CAD build for the part. Positions are in the model's coordinates, mm. A direction names the side the tool comes from. Round coordinates to 2 decimals unless told otherwise and drop trailing zeros. Write each loop counter-clockwise with the first axis right and the second up, starting at its lowest first coordinate (ties: lowest second). Pieces come first, ordered by that corner, then holes. Notation, with made-up numbers: (89, 71.25) - (126, 71.25) arc R16 ccw to (126, 77.25) - close; hole circle Ø8 at (-34, 81). An arc over 180 degrees is marked (long way). Put each result on its own line as item: value. Start each with the question number.
Item 1: Cut at C-C (z = 12.75). Give the cut face in (x, y).
Item 2: Cut at A-A (x = 40). Give the cut face in (y, z), and give its area (3 significant figures).
Item 3: 3-axis set-ups, long thin cutter, end or side, ignore diameter. For faces 1 (the cylindrical face through (9.1, 19.5, 8.8)), 2 (the flat face through (49, 10, 1)): which of +Z, -Z, +X, -X, +Y, -Y reach the whole face in a straight line?
Item 4: Pin check, flat tip, straight feed: pin 1 Ø5 at (x, z) = (30, 10) entering from +Y. Stop position of the tip, or through.
Item 5: Mould opens along Z. For faces 3 (the cylindrical face through (86.15, 15.07, 0.51)), 4 (the cylindrical face through (61.487, 19.507, 9.805)) say: released by +Z, released by -Z, zero draft, split by the parting line, or undercut.
Item 6: Cut at B-B (y = 5). Give the cut face in (x, z), and give its area (3 significant figures).
Item 7: Drill centre lines: line 1 (Y direction, x = 87.65, z = 19.45); line 2 (Y direction, x = 25.5, z = 7.5). Where is each one in solid material? Low to high. Write a range as from..to.
```python
from build123d import *

# Parameters (mm, degrees)
SKETCH_1_W          = 20
SKETCH_1_H          = 20
SKETCH_1_W_2        = 18
SKETCH_1_H_2        = 18
EXTRUDE_1_DEPTH     = 100
SKETCH_2_R          = 1.5
CUT_EXTRUDE_1_DEPTH = 104.923048454
SKETCH_3_R          = 1.5
CUT_EXTRUDE_2_DEPTH = 104.923048454


with BuildPart() as part:
    # 草图1 → 凸台-拉伸1 (new body)
    with BuildSketch(Plane(origin=(0, 0, 0), x_dir=(0, 0, -1), z_dir=(1, 0, 0))):
        with Locations((-10, 10)):
            Rectangle(SKETCH_1_W, SKETCH_1_H)
        with Locations((-10, 10)):
            Rectangle(SKETCH_1_W_2, SKETCH_1_H_2, mode=Mode.SUBTRACT)
    extrude(amount=EXTRUDE_1_DEPTH)

    # 草图2 → 切除-拉伸1 (cut, through all)
    with BuildSketch(Plane.XY.offset(20)):
        with Locations((72.65, 15)):
            Circle(SKETCH_2_R)
        with Locations(Location((72.65, 5, 0), (0, 0, 180))):
            Circle(SKETCH_2_R)
        with Locations((87.65, 15)):
            Circle(SKETCH_2_R)
        with Locations(Location((87.65, 5, 0), (0, 0, 180))):
            Circle(SKETCH_2_R)
    extrude(amount=-CUT_EXTRUDE_1_DEPTH, mode=Mode.SUBTRACT)

    # 草图3 → 切除-拉伸2 (cut, through all)
    with BuildSketch(Plane(origin=(0, 20, 0), x_dir=(1, 0, 0), z_dir=(0, 1, 0))):
        with Locations(Location((90, -10, 0), (0, 0, 270))):
            Circle(SKETCH_3_R)
        with Locations(Location((80, -10, 0), (0, 0, 270))):
            Circle(SKETCH_3_R)
        with Locations(Location((70, -10, 0), (0, 0, 270))):
            Circle(SKETCH_3_R)
        with Locations(Location((60, -10, 0), (0, 0, 270))):
            Circle(SKETCH_3_R)
        with Locations(Location((50, -10, 0), (0, 0, 270))):
            Circle(SKETCH_3_R)
        with Locations(Location((40, -10, 0), (0, 0, 270))):
            Circle(SKETCH_3_R)
        with Locations(Location((30, -10, 0), (0, 0, 270))):
            Circle(SKETCH_3_R)
        with Locations(Location((20, -10, 0), (0, 0, 270))):
            Circle(SKETCH_3_R)
        with Locations(Location((10, -10, 0), (0, 0, 270))):
            Circle(SKETCH_3_R)
    extrude(amount=-CUT_EXTRUDE_2_DEPTH, mode=Mode.SUBTRACT)


solid = part.part
```
Output values:
1. outline: (0, 0) - (100, 0) - (100, 1) - (0, 1) - close; (0, 19) - (100, 19) - (100, 20) - (0, 20) - close
2. outline: (0, 0) - (20, 0) - (20, 8.5) - (19, 8.5) - (19, 1) - (1, 1) - (1, 8.5) - (0, 8.5) - close; (0, 11.5) - (1, 11.5) - (1, 19) - (19, 19) - (19, 11.5) - (20, 11.5) - (20, 20) - (0, 20) - close
2. area: 70.0 mm2
3. face 1: +Y, -Y
3. face 2: +X, -X
4. pin 1: y = 20
5. face 3: zero draft
5. face 4: undercut
6. outline: (0, 0) - (71.15, 0) - (71.15, 1) - (0, 1) - close; (0, 19) - (71.15, 19) - (71.15, 20) - (0, 20) - close; (74.15, 0) - (86.15, 0) - (86.15, 1) - (74.15, 1) - close; (74.15, 19) - (86.15, 19) - (86.15, 20) - (74.15, 20) - close; (89.15, 0) - (100, 0) - (100, 1) - (89.15, 1) - close; (89.15, 19) - (100, 19) - (100, 20) - (89.15, 20) - close
6. area: 188 mm2
7. line 1: 0..3.5, 6.5..13.5, 16.5..20
7. line 2: 0..1, 19..20
